Check sheet for the modelled part. Datum: model origin and axes. Units: mm. A direction names the side the tool comes from. Give positions to 0.01 mm unless a question says otherwise; leave off trailing zeros. Write each loop counter-clockwise with the first axis right and the second up, starting at its lowest first coordinate (ties: lowest second). Pieces come first, ordered by that corner, then holes. Notation, with made-up numbers: (-1.75, 56) - (20.25, 56) arc R9 ccw to (20.25, 72) - close; hole circle Ø5 at (47, 81). An arc over 180 degrees is marked (long way). Return JSON: item names as keys, results as strings. Group by question number.
Autodesk Fusion 360 part; units mm, degrees
sketch "Sketch1" plane through (0, 0, 0) normal (0, 0, 1) x (1, 0, 0)
  line L0 (0, 0) -> (61, 0)
  line L1 (61, 0) -> (61, 49)
  line L2 (61, 49) -> (0, 49)
  line L3 (0, 49) -> (0, 0)
  line L4 (16, 10) -> (25, 10)
  line L5 (25, 10) -> (25, 6.3)
  line L6 (25, 6.3) -> (16, 6.3)
  line L7 (16, 6.3) -> (16, 10)
  line L8 (45, 18) -> (54.5, 18)
  line L9 (54.5, 18) -> (54.5, 6.5)
  line L10 (54.5, 6.5) -> (45, 6.5)
  line L11 (45, 6.5) -> (45, 18)
  dimension "d1" = 61
  dimension "d2" = 49
  dimension "d3" = 9
  dimension "d4" = 3.7
  dimension "d5" = 10
  dimension "d6" = 16
  dimension "d7" = 9.5
  dimension "d8" = 11.5
  dimension "d9" = 45
  dimension "d10" = 18
extrude "Extrude1" add sketch "Sketch1" along normal blind 1.5
fillet "Fillet1" radius 2 4 edges at (0, 0, 0.75) (61, 0, 0.75) (61, 49, 0.75) (0, 49, 0.75)
Item 1: Section check A-A on x = 47.5. Record the cut outline in (y, z), plus the area to 4 significant figures.
Item 2: Access from +Z, -Z, +X, -X, +Y, -Y to the whole of each face (thin tool, end or side, straight path). Record for faces 4 (the face through (30, 25, 1.5)), 5 (the face through (16, 8, 1)).
Item 3: Section check B-B on y = 8.5. Record the cut outline in (x, z).
Item 4: Mould release check, pull along X, two halves, no side actions. Record for faces 1 (the face through (61, 24, 1)), 2 (the face through (0, 25, 1)), 3 (the face through (20, 10, 1)): +X half, -X half, draft (parallel to the pull), parting line (faces both ways), or undercut.
Item 5: Material ranges on line 1 along Y through (x, z) = (22, 0.3), recorded low to high. Write a range as from..to.
Item 6: Section check C-C on z = 1.05. Record the cut outline in (x, y), plus the area to 3 significant figures.
Reply:
{
 "1": {"outline": "(0, 0) - (6.5, 0) - (6.5, 1.5) - (0, 1.5) - close; (18, 0) - (49, 0) - (49, 1.5) - (18, 1.5) - close", "area": "56.25 mm²"},
 "2": {"face 4": "+Z, +X, -X, +Y, -Y", "face 5": "+Z, -Z"},
 "3": {"outline": "(0, 0) - (16, 0) - (16, 1.5) - (0, 1.5) - close; (25, 0) - (45, 0) - (45, 1.5) - (25, 1.5) - close; (54.5, 0) - (61, 0) - (61, 1.5) - (54.5, 1.5) - close"},
 "4": {"face 1": "+X half", "face 2": "-X half", "face 3": "undercut"},
 "5": {"line 1": "0..6.3, 10..49"},
 "6": {"outline": "(0, 2) arc R2 ccw to (2, 0) - (59, 0) arc R2 ccw to (61, 2) - (61, 47) arc R2 ccw to (59, 49) - (2, 49) arc R2 ccw to (0, 47) - close; hole (16, 6.3) - (25, 6.3) - (25, 10) - (16, 10) - close; hole (45, 6.5) - (54.5, 6.5) - (54.5, 18) - (45, 18) - close", "area": "2,840 mm²"}
}
